from build123d import *

# Parameters (mm, degrees)
PAD014_DEPTH       = 6.5
POLARPATTERN_COUNT = 19
PAD015_DEPTH       = 8.5


with BuildPart() as part:
    # Sketch031 → Revolution002 (revolve)
    with BuildSketch(Plane.YZ):
        Polygon((2.5, 0), (7.03, 0), (7.03, 1), (6.03, 1), (6.03, 7.5), (7.03, 7.5), (7.03, 8.5), (2.5, 8.5), align=None)
    revolve(axis=Axis((0, 0, 0), (0, 0, 1)))

    # Sketch029 → Pad014 (new body)
    with BuildSketch(Plane.XY.offset(1)):
        with BuildLine():
            ThreePointArc((5.78, -0.433013), (6.53, 0), (5.78, 0.433013))
            Line((5.78, 0.433013), (5.78, -0.433013))
        make_face()
    pad014 = extrude(amount=PAD014_DEPTH)

    # PolarPattern: Pad014 ×19 about axis
    polarpattern_axis = Axis((0, 0, 1), (0, 0, 1))
    for i in range(1, POLARPATTERN_COUNT):
        add(pad014.rotate(polarpattern_axis, i * 360 / POLARPATTERN_COUNT))

    # Sketch032 → Pad015 (join)
    with BuildSketch(Plane.XY):
        with BuildLine():
            ThreePointArc((2, -1.5), (2.5, 0), (2, 1.5))
            Line((2, 1.5), (2, -1.5))
        make_face()
    extrude(amount=PAD015_DEPTH)


solid = part.part
Verification items for the finished model (mm, model axes). A direction names the side the tool comes from. Give positions to 0.01 mm unless a question says otherwise; leave off trailing zeros. Loops run counter-clockwise (first coordinate to the right, second up) from the corner with the lowest first, then second, coordinate; pieces in that order, holes last. Notation, with made-up numbers: (53, -20) - (104, -20) arc R24 cw to (104, 19) - close; hole circle Ø6 at (51.5, 32.5). An arc over 180 degrees is marked (long way). Write each question's results on one line, items separated by ' | '.
1) Sectioned sample at A-A on y = 0. Record the boundary of the cut face in (x, z).
Solution:
outline: (-7.03, 0) - (-2.5, 0) - (-2.5, 8.5) - (-7.03, 8.5) - (-7.03, 7.5) - (-6.03, 7.5) - (-6.03, 1) - (-7.03, 1) - close; (2, 0) - (7.03, 0) - (7.03, 1) - (6.53, 1) - (6.53, 7.5) - (7.03, 7.5) - (7.03, 8.5) - (2, 8.5) - close
2) Depth check by flat-ended pin: P1, Ø1.5, axis at x = -1.5, z = 7, coming from the +Y side; P2, Ø1, axis at x = 1, y = -4, coming from the -Z side; P3, Ø0.9, axis at y = 0.5, z = 4, coming from the -X side; P4, Ø1, axis at x = -2.5, z = 4, coming from the +Y side. Enter the tip coordinate at first touch or a pass-through.
Solution:
P1: y = 6.97 | P2: z = 0 | P3: x = -6.45 | P4: y = 6.02
3) Sectioned sample at B-B on x = -3.25. Record the boundary of the cut face in (y, z).
Solution:
outline: (-6.23, 0) - (6.23, 0) - (6.23, 1) - (5.08, 1) - (5.08, 7.5) - (6.23, 7.5) - (6.23, 8.5) - (-6.23, 8.5) - (-6.23, 7.5) - (-5.08, 7.5) - (-5.08, 1) - (-6.23, 1) - close
4) Sectioned sample at C-C on y = -2.75. Record the boundary of the cut face in (x, z), plus the area to 3 significant figures.
Solution:
outline: (-6.47, 0) - (6.47, 0) - (6.47, 1) - (5.37, 1) - (5.37, 7.5) - (6.47, 7.5) - (6.47, 8.5) - (-6.47, 8.5) - (-6.47, 7.5) - (-5.79, 7.5) - (-5.79, 1) - (-6.47, 1) - close | area: 98.4 mm2
5) Material ranges on L1, parallel to X at y = 0, z = 6.75; L2, parallel to Z at x = 6, y = -3.25; L3, parallel to X at y = 1, z = 2.75, recorded low to high. Write a range as from..to.
Solution:
L1: -6.03..-2.5, 2..6.53 | L2: 0..1, 7.5..8.5 | L3: -6.45..-2.29, 2..5.95
6) Tool access check on faces 1 (the flat face through (0, -3, 0)), 2 (the cylindrical face through (-4.414, 4.812, 4.204)), 3 (the cylindrical face through (5.95, 0.99, 4.3)), 4 (the flat face through (2, 0, 4)). Record the directions out of +Z, -Z, +X, -X, +Y, -Y that give a thin tool (end or side, any length) a straight path to the whole face; none if there is none.
Solution:
face 1: -Z, +X, -X, +Y, -Y | face 2: none | face 3: +X | face 4: +Z, -Z
7) Mould release check, pull along Y, two halves, no side actions. Record for faces 5 (the flat face through (0, 3, 8.5)), 6 (the cylindrical face through (-1.487, -5.844, 4.296)), 7 (the cylindrical face through (0.5, 6.01, 4.3)), 8 (the cylindrical face through (5.16, 4, 4.2)): pulls with the +Y half, pulls with the -Y half, needs draft (parallel to the pull), parting line crosses it, or undercut.
Solution:
face 5: needs draft | face 6: pulls with the -Y half | face 7: pulls with the +Y half | face 8: undercut
